from build123d import *

# Parameters (mm, degrees)
F1_DEPTH = 5
F2_W     = 10
F2_H     = 5
F3_DEPTH = 6
F2_W_2   = 5
F2_H_2   = 10


with BuildPart() as f1:
    # F0 (on Top) → F1 (new body)
    with BuildSketch(Plane.XY):
        with BuildLine():
            ThreePointArc((0, 5), (1.4644660941, 1.4644660941), (5, 0))
            Line((5, 0), (38.87, 0))
            ThreePointArc((38.87, 0), (42.4055339059, 1.4644660941), (43.87, 5))
            Line((43.87, 5), (43.87, 49.36))
            Line((43.87, 49.36), (43.87, 65.05))
            ThreePointArc((43.87, 65.05), (42.4055339059, 68.5855339059), (38.87, 70.05))
            Line((38.87, 70.05), (5, 70.05))
            ThreePointArc((5, 70.05), (1.4644660941, 68.5855339059), (0, 65.05))
            Line((0, 65.05), (0, 5))
        make_face()
        with BuildLine():
            ThreePointArc((9.82, 12.55), (8.1128932188, 11.8428932188), (8.82, 13.55))
            ThreePointArc((8.82, 13.55), (9.5271067812, 13.2571067812), (9.82, 12.55))
        make_face(mode=Mode.SUBTRACT)
        with BuildLine():
            ThreePointArc((8.82, 26.55), (7.82, 27.55), (8.82, 28.55))
            ThreePointArc((8.82, 28.55), (9.5271067812, 28.2571067812), (9.82, 27.55))
            ThreePointArc((9.82, 27.55), (9.5271067812, 26.8428932188), (8.82, 26.55))
        make_face(mode=Mode.SUBTRACT)
        with BuildLine():
            ThreePointArc((28.42, 49.36), (29.42, 50.36), (30.42, 49.36))
            ThreePointArc((30.42, 49.36), (29.42, 48.36), (28.42, 49.36))
        make_face(mode=Mode.SUBTRACT)
    extrude(amount=F1_DEPTH)

    # F2 (on face) → F3, piece 2 (join)
    with BuildSketch(Plane.XY.offset(5)):
        with Locations((41.37, 10)):
            Rectangle(F2_W_2, F2_H_2)
        with Locations((2.5, 60.05)):
            Rectangle(F2_W_2, F2_H_2)
    extrude(amount=F3_DEPTH)


with BuildPart() as f3:
    # F2 (on face) → F3 (new body)
    with BuildSketch(Plane.XY.offset(5)):
        with Locations((33.87, 2.5)):
            Rectangle(F2_W, F2_H)
    extrude(amount=F3_DEPTH)


solid = f1.part
Can you work these out from the model? Positions are in its coordinate system, mm. A direction names the side the tool comes from. Give positions to 0.01 mm unless a question says otherwise; leave off trailing zeros. Order: outer loops, then holes, each group sorted by start corner. A loop starts at its lowest first (then second) coordinate and runs counter-clockwise, first axis right, second up. Notation, with made-up numbers: M 45,58.5 L 85,58.5 A23 cw 85,80.5 Z; hole C -31,-13 d6. An arc over 180 degrees is marked long. Use one line per item in the form item = value.
Item 1: For faces 1 (the flat face through (41, 5, 8)), 2 (the flat face through (2, 65.05, 8)), 3 (the flat face through (5, 60, 8)), which set-ups out of +Z, -Z, +X, -X, +Y, -Y let a thin tool reach every point of the face, with its end or its side?
Values follow:
face_1 = +Z, +X, -X, -Y
face_2 = +Z, +X, -X, +Y
face_3 = +Z, +X, +Y, -Y
Item 2: If we section it at A-A, the plane z = 10: Write out the boundary of the cut face in (x, y), and give its area (3 significant figures).
Values follow:
outline = M 0,55.05 L 5,55.05 L 5,65.05 L 0,65.05 Z; M 38.87,5 L 43.87,5 L 43.87,15 L 38.87,15 Z
area = 100 mm^2
Item 3: Thinking about a two-plate mould opening in X: for faces 4 (the flat face through (2, 55.05, 8)), 5 (the cylindrical face through (30.374, 49.06, 2.465)), 6 (the flat face through (38.87, 10, 8)), which applies, pulls with the +X half, pulls with the -X half, needs draft (parallel to the pull), parting line crosses it, or undercut?
Values follow:
face_4 = needs draft
face_5 = undercut
face_6 = pulls with the -X half
Item 4: If we section it at D-D, the plane x = 26.5: Write out the boundary of the cut face in (y, z).
Values follow:
outline = M 0,0 L 70.05,0 L 70.05,5 L 0,5 Z
Item 5: If I drill on line 1 along Y through (x, z) = (8.82, 1.2); line 2 along Y through (x, z) = (29.42, 1.9); line 3 along X through (y, z) = (12.55, 3.9), over which ranges is the centre line in solid material (lowest first)? Write a range as [from, to].
Values follow:
line_1 = [0, 11.55], [13.55, 26.55], [28.55, 70.05]
line_2 = [0, 48.36], [50.36, 70.05]
line_3 = [0, 7.82], [9.82, 43.87]
Item 6: If we section it at C-C, the plane y = 57.5: Write out the boundary of the cut face in (x, z), and give its area (3 significant figures).
Values follow:
outline = M 0,0 L 43.87,0 L 43.87,5 L 5,5 L 5,11 L 0,11 Z
area = 249 mm^2
Item 7: If we section it at B-B, the plane y = 49.36: Write out the boundary of the cut face in (x, z).
Values follow:
outline = M 0,0 L 28.42,0 L 28.42,5 L 0,5 Z; M 30.42,0 L 43.87,0 L 43.87,5 L 30.42,5 Z
Item 8: Will these pins go through, and if not, where does the flat tip stop? pin 1 Ø4 at (x, z) = (25, 8) entering from +Y; pin 2 Ø5.5 at (x, z) = (42, 8) entering from +Y; pin 3 Ø4 at (x, z) = (3.5, 9) entering from -Y; pin 4 Ø22 at (x, y) = (23.5, 52) entering from +Z.
Values follow:
pin_1 = through
pin_2 = 15
pin_3 = 55.05
pin_4 = 5
